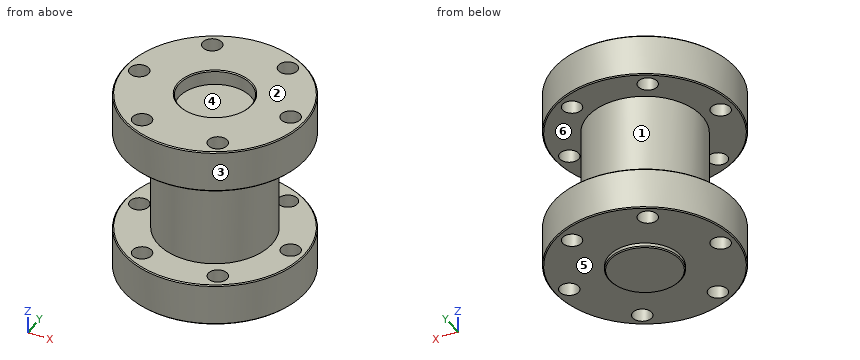
```python
from build123d import *

# Parameters (mm, degrees)
F0_R      = 68.2625
F0_R_2    = 7.14375
F1_DEPTH  = 31.75
F3_R      = 68.2625
F3_R_2    = 7.14375
F4_DEPTH  = 31.75
F5_R      = 42.8625
F6_DEPTH  = 81.28
F7_R      = 27.051
F8_DEPTH  = 11.1125
F9_R      = 26.9875
F10_DEPTH = 3.175
F11_SIZE  = 0.762


with BuildPart() as f1:
    # F0 (on Top) → F1 (new body)
    with BuildSketch(Plane.XY):
        Circle(F0_R)
        with Locations((-28.575, -49.493352)):
            Circle(F0_R_2, mode=Mode.SUBTRACT)
        with Locations((28.575, -49.493352)):
            Circle(F0_R_2, mode=Mode.SUBTRACT)
        with Locations((-57.15, 0)):
            Circle(F0_R_2, mode=Mode.SUBTRACT)
        with Locations((-28.575, 49.493352)):
            Circle(F0_R_2, mode=Mode.SUBTRACT)
        with Locations((57.15, 0)):
            Circle(F0_R_2, mode=Mode.SUBTRACT)
        with Locations((28.575, 49.493352)):
            Circle(F0_R_2, mode=Mode.SUBTRACT)
    extrude(amount=F1_DEPTH)



with BuildPart() as f4:
    # F3 (on offset) → F4 (new body)
    with BuildSketch(Plane.XY.offset(-107.95)):
        Circle(F3_R)
        with Locations((-28.575, -49.493352)):
            Circle(F3_R_2, mode=Mode.SUBTRACT)
        with Locations((28.575, -49.493352)):
            Circle(F3_R_2, mode=Mode.SUBTRACT)
        with Locations((-57.15, 0)):
            Circle(F3_R_2, mode=Mode.SUBTRACT)
        with Locations((-28.575, 49.493352)):
            Circle(F3_R_2, mode=Mode.SUBTRACT)
        with Locations((57.15, 0)):
            Circle(F3_R_2, mode=Mode.SUBTRACT)
        with Locations((28.575, 49.493352)):
            Circle(F3_R_2, mode=Mode.SUBTRACT)
    extrude(amount=F4_DEPTH)


with BuildPart() as f1_1:
    add(f1.part)

    add(f4.part)  # F6 merges F4
    # F5 (on face) → F6 (join)
    with BuildSketch(Plane(origin=(0, 0, 0), x_dir=(1, 0, 0), z_dir=(0, 0, -1))):
        Circle(F5_R)
    extrude(amount=F6_DEPTH)

    # F7 (on face) → F8 (cut)
    with BuildSketch(Plane.XY.offset(31.75)):
        Circle(F7_R)
    extrude(amount=-F8_DEPTH, mode=Mode.SUBTRACT)

    # F9 (on face) → F10 (join)
    with BuildSketch(Plane(origin=(0, 0, -107.95), x_dir=(1, 0, 0), z_dir=(0, 0, -1))):
        Circle(F9_R)
    extrude(amount=F10_DEPTH)

    # F11
    f11_edges = [f1_1.edges().sort_by_distance(p)[0] for p in [
        (-68.2625, 0, 31.75),
        (-27.051, 0, 31.75),
        (-68.2625, 0, 0),
        (-68.2625, 0, -76.2),
        (-68.2625, 0, -107.95),
        (-26.9875, 0, -111.125),
    ]]
    chamfer(f11_edges, length=F11_SIZE)


solid = f1_1.part
```
Design review of the part built by this model. Coordinates are the model's own, in mm. Face numbers are marked on the shaded views. A direction names the side the tool comes from. Round coordinates to 2 decimals unless told otherwise and drop trailing zeros. Write each loop counter-clockwise with the first axis right and the second up, starting at its lowest first coordinate (ties: lowest second). Pieces come first, ordered by that corner, then holes. Notation, with made-up numbers: (12.5, 70) -> (50.5, 70) arc R31 ccw to (50.5, 108) -> close; hole circle Ø7 at (-16.75, -18.75). An arc over 180 degrees is marked (long way). Write item = value, one per line. Start each with the question number.
1) Take a section at B-B, the plane y = 0. Count the separate pieces of the cut face and the enclosed holes in it, plus the area to 3 significant figures.
2) Clearance check with flat-ended pins moving along their axes: pin 1 (23 mm diameter, centred on x = -28.58, y = -49.49, fed in from -Z); pin 2 (23 mm diameter, centred on x = 28.58, y = -49.49, fed in from +Z); pin 3 (13 mm diameter, centred on x = 28.58, y = 49.49, fed in from -Z); pin 4 (12 mm diameter, centred on y = 11.5, z = -57.5, fed in from -X). State where each tip first meets the part, or that it passes through.
3) Tool access review of the marked faces 1 and 2: name each direction out of +Z, -Z, +X, -X, +Y, -Y from which nothing blocks a thin tool from reaching the whole face with its end or side.
4) Wall thickness on probe 1 along X at (y, z) = (-1.5, -96); probe 2 along Z at (x, y) = (44.5, 8); probe 3 along X at (y, z) = (55, 13): over which ranges is each line inside the solid? List them lowest first. Write a range as from..to.
5) Take a section at C-C, the plane z = -3.5. State the section outline as (x, y) points (1 decimal).
6) Mouldability with a two-part tool opening along Z and no side actions: class the marked faces 3, 4, 5 and 6 as +Z half, -Z half, draft (parallel to the pull), parting line (faces both ways), or undercut.
Results list:
q1.separate_pieces = 5
q1.enclosed_holes = 0
q1.area = 13,000 mm²
q2.pin_1 = -107.95
q2.pin_2 = 31.75
q2.pin_3 = through
q2.pin_4 = -42.51
q3.face_1 = none
q3.face_2 = +Z, +X, -X, +Y, -Y
q4.probe_1 = -68.25..-64.13, -50.17..50.17, 64.13..68.25
q4.probe_2 = -107.95..-76.2, 0..31.75
q4.probe_3 = -40.43..-33.13, -24.02..24.02, 33.13..40.43
q5.outline = circle Ø85.7 at (0, 0)
q6.face_3 = draft
q6.face_4 = +Z half
q6.face_5 = -Z half
q6.face_6 = undercut
